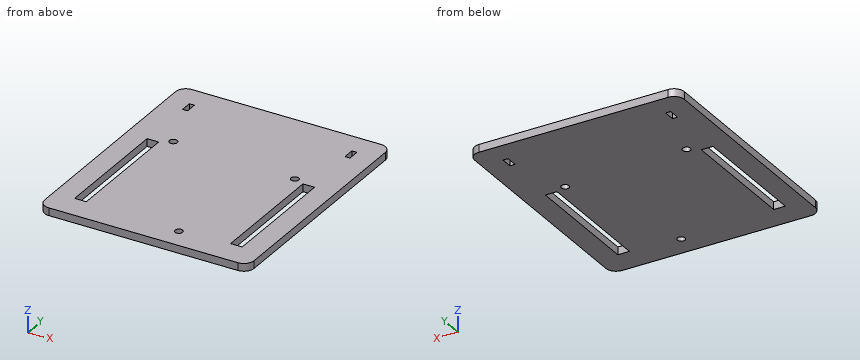
from build123d import *

# Parameters (mm, degrees)
ESQUISSE1_R        = 1.5
ESQUISSE1_R_2      = 1.548892625
ESQUISSE1_W        = 4.54
ESQUISSE1_H        = 47.72
ESQUISSE1_W_2      = 1.965612554
ESQUISSE1_H_2      = 4.508607734
BOSS_EXTRU_1_DEPTH = 3
CONG_1_R           = 4


with BuildPart() as part:
    # Esquisse1 → Boss.-Extru.1 (new body)
    with BuildSketch(Plane.XY):
        Polygon((-41.006346513, 88.5), (41.006346513, 88.5), (41.006346513, -6), (-40.884024197, -6), align=None)
        with Locations((8.896346513, 2.5)):
            Circle(ESQUISSE1_R, mode=Mode.SUBTRACT)
        with Locations((-24.123653487, 54.57)):
            Circle(ESQUISSE1_R_2, mode=Mode.SUBTRACT)
        with Locations((24.136346513, 53.3)):
            Circle(ESQUISSE1_R, mode=Mode.SUBTRACT)
        with Locations((-30.473653487, 27.9)):
            Rectangle(ESQUISSE1_W, ESQUISSE1_H, mode=Mode.SUBTRACT)
        with Locations((30.486346513, 27.9)):
            Rectangle(ESQUISSE1_W, ESQUISSE1_H, mode=Mode.SUBTRACT)
        with Locations((31.773540236, 77.411308687)):
            Rectangle(ESQUISSE1_W_2, ESQUISSE1_H_2, mode=Mode.SUBTRACT)
        with Locations((-31.773540236, 77.411308687)):
            Rectangle(ESQUISSE1_W_2, ESQUISSE1_H_2, mode=Mode.SUBTRACT)
    extrude(amount=BOSS_EXTRU_1_DEPTH)

    # Congé1
    cong_1_edges = [part.edges().sort_by_distance(p)[0] for p in [
        (-41.006346513, 88.5, 1.5),
        (41.006346513, 88.5, 1.5),
        (41.006346513, -6, 1.5),
        (-40.884024197, -6, 1.5),
    ]]
    fillet(cong_1_edges, radius=CONG_1_R)


solid = part.part
Could you check a few things on this model? Use its own coordinates, in mm. Coordinates: 2 decimals unless noted, no trailing zeros. Write each loop counter-clockwise with the first axis right and the second up, starting at its lowest first coordinate (ties: lowest second). Pieces come first, ordered by that corner, then holes. Notation, with made-up numbers: (19, -14.5) - (44, -14.5) arc R20 ccw to (44, -3.5) - close; hole circle Ø4 at (75, -11.5). An arc over 180 degrees is marked (long way). Write item = value, one per line.
1) Will these pins go through, and if not, where does the flat tip stop? pin 1 Ø1.8 at (x, y) = (8.9, 2.5) entering from +Z (3 decimals); pin 2 Ø1.5 at (y, z) = (77, 1.5) entering from -X; pin 3 Ø1.5 at (y, z) = (24, 1.5) entering from -X.
Result set:
pin_1 = through
pin_2 = -40.99
pin_3 = -40.92
2) Suppose I cut it at D-D on y = 46. Please give me the cut outline in (x, z), plus the area to 3 significant figures.
Result set:
outline = (-40.95, 0) - (-32.74, 0) - (-32.74, 3) - (-40.95, 3) - close; (-28.2, 0) - (28.22, 0) - (28.22, 3) - (-28.2, 3) - close; (32.76, 0) - (41.01, 0) - (41.01, 3) - (32.76, 3) - close
area = 219 mm2
3) Please list where these lines run through material, in increasing order: line 1 (X direction, y = 9, z = 0.8); line 2 (X direction, y = 45.5, z = 2); line 3 (X direction, y = 65, z = 0.6). Write a range as [from, to].
Result set:
line_1 = [-40.9, -32.74], [-28.2, 28.22], [32.76, 41.01]
line_2 = [-40.95, -32.74], [-28.2, 28.22], [32.76, 41.01]
line_3 = [-40.98, 41.01]
4) Suppose I cut it at A-A on z = 1.4. Please give me the cut outline in (x, y).
Result set:
outline = (-41, 84.49) - (-40.89, -2.01) arc R4 ccw to (-36.89, -6) - (37.01, -6) arc R4 ccw to (41.01, -2) - (41.01, 84.5) arc R4 ccw to (37.01, 88.5) - (-37, 88.5) arc R4 ccw to start; hole (-32.76, 75.16) - (-30.79, 75.16) - (-30.79, 79.67) - (-32.76, 79.67) - close; hole (-32.74, 4.04) - (-28.2, 4.04) - (-28.2, 51.76) - (-32.74, 51.76) - close; hole circle Ø3.1 at (-24.12, 54.57); hole circle Ø3 at (8.9, 2.5); hole circle Ø3 at (24.14, 53.3); hole (28.22, 4.04) - (32.76, 4.04) - (32.76, 51.76) - (28.22, 51.76) - close; hole (30.79, 75.16) - (32.76, 75.16) - (32.76, 79.67) - (30.79, 79.67) - close
5) Suppose I cut it at B-B on y = 2.5. Please give me the cut outline in (x, z), plus the area to 3 significant figures.
Result set:
outline = (-40.9, 0) - (7.4, 0) - (7.4, 3) - (-40.9, 3) - close; (10.4, 0) - (41.01, 0) - (41.01, 3) - (10.4, 3) - close
area = 237 mm2
6) Suppose I cut it at C-C on y = 19.5. Please give me the cut outline in (x, z).
Result set:
outline = (-40.92, 0) - (-32.74, 0) - (-32.74, 3) - (-40.92, 3) - close; (-28.2, 0) - (28.22, 0) - (28.22, 3) - (-28.2, 3) - close; (32.76, 0) - (41.01, 0) - (41.01, 3) - (32.76, 3) - close
